The model under review builds one solid part; all positions refer to its coordinate system, in mm. Face numbers are marked on the shaded views. Coordinates: 2 decimals unless noted, no trailing zeros. Write each loop counter-clockwise with the first axis right and the second up, starting at its lowest first coordinate (ties: lowest second). Pieces come first, ordered by that corner, then holes. Notation, with made-up numbers: (54, -32) - (72, -32) arc R25 ccw to (72, -5) - close; hole circle Ø9 at (54.25, 62.25). An arc over 180 degrees is marked (long way). Return JSON: item names as keys, results as strings. Group by question number.
(1) We need section C-C on x = -11.5. State the section outline as (y, z) points, then the cut area to 3 significant figures.
(2) We need section A-A on z = -0.3. State the section outline as (x, y) points, then the cut area to 3 significant figures.
(3) We need section B-B on x = -3. State the section outline as (y, z) points, then the cut area to 3 significant figures.
(4) To check wall thickness, follow L1, parallel to X at y = 11.75, z = -0.1; L2, parallel to Y at x = -13, z = -0.55; L3, parallel to Y at x = 6, z = 0.5. State the ranges of each line that lie inside material, in increasing order. Write a range as from..to.
(5) For pin 1 Ø1.5 at (x, z) = (-0.5, -0.5) entering from +Y, flat-tipped, find the tip position at first contact; note if it passes through.
(6) Draft analysis for pull direction X (two halves, no side actions). For the marked faces 1, 2 and 3, state which applies: released by +X, released by -X, zero draft, split by the parting line, or undercut.
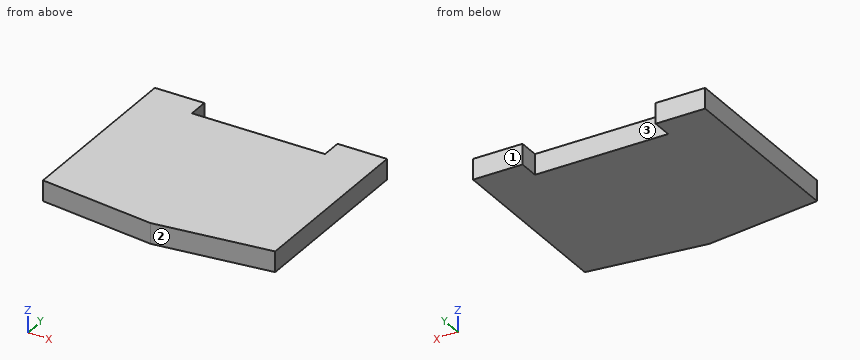
Autodesk Inventor part; units mm, degrees
ref_plane "YZ Plane" through (0, 0, 0) normal (1, 0, 0) x (0, 1, 0)
ref_plane "XZ Plane" through (0, 0, 0) normal (0, 1, 0) x (-1, 0, 0)
ref_plane "XY Plane" through (0, 0, 0) normal (0, 0, 1) x (1, 0, 0)
sketch "Sketch1" plane through (0, 0, 0) normal (0, 0, 1) x (1, 0, 0)
  line L0 (-17, 14.5) -> (17, 14.5)
  line L1 (17, 14.5) -> (17, -14.5)
  line L2 (17, -14.5) -> (-17, -14.5)
  line L3 (-17, -14.5) -> (-17, 14.5)
  line L4 (-9.75, 14.5) -> (9.75, 14.5)
  line L5 (9.75, 14.5) -> (9.75, 11.5)
  line L6 (9.75, 11.5) -> (-9.75, 11.5)
  line L7 (-9.75, 11.5) -> (-9.75, 14.5)
  line L8 (0, -14.5) -> (0, -12.42)
  line L9 (17, -12.42) -> (0, -14.5)
  line L10 (0, -14.5) -> (-17, -12.42)
  point P0 (0, 0)
  point P1 (17, 0)
  point P2 (0, 14.5)
  point P3 (9.75, 14.5)
  dimension "d0" = 34
  dimension "d1" = 29
  dimension "d3" = 2.08
  dimension "d6" = 19.5
  dimension "d7" = 3
extrude "Extrusion1" add sketch "Sketch1" along normal mid plane 3 contours L0 L7 L6 L5 L1 L9 L10 L3
properties part number "A"
Ans:
{
 "1": {"outline": "(-13.09, -1.5) - (14.5, -1.5) - (14.5, 1.5) - (-13.09, 1.5) - close", "area": "82.8 mm²"},
 "2": {"outline": "(-17, -12.42) - (0, -14.5) - (17, -12.42) - (17, 14.5) - (9.75, 14.5) - (9.75, 11.5) - (-9.75, 11.5) - (-9.75, 14.5) - (-17, 14.5) - close", "area": "892 mm²"},
 "3": {"outline": "(-14.13, -1.5) - (11.5, -1.5) - (11.5, 1.5) - (-14.13, 1.5) - close", "area": "76.9 mm²"},
 "4": {"L1": "-17..-9.75, 9.75..17", "L2": "-12.91..14.5", "L3": "-13.77..11.5"},
 "5": {"pin 1": "y = 11.5"},
 "6": {"face 1": "zero draft", "face 2": "released by +X", "face 3": "undercut"}
}
